```python
from build123d import *

# Parameters (mm, degrees)
SKETCH_1_R      = 2.5
EXTRUDE_1_DEPTH = 3


with BuildPart() as part:
    # 草图1 → 凸台-拉伸1 (new body)
    with BuildSketch(Plane(origin=(0, 0, 0), x_dir=(1, 0, 0), z_dir=(0, 1, 0))):
        with BuildLine():
            ThreePointArc((19, -6), (24.605034154, -2.140932539), (23, 4.472135955))
            Line((23, 4.472135955), (23, 10))
            ThreePointArc((23, 10), (19, 14), (15, 10))
            Line((15, 10), (15, 6))
            Line((15, 6), (0, 6))
            ThreePointArc((0, 6), (-6, 0), (0, -6))
            Line((0, -6), (19, -6))
        make_face()
        with BuildLine():
            ThreePointArc((0.315789474, -3.987515142), (-4, 0), (0.315789474, 3.987515142))
            Line((0.315789474, 3.987515142), (19.197368421, 2.492196964))
            ThreePointArc((19.197368421, 2.492196964), (21.5, 0), (19.197368421, -2.492196964))
            Line((19.197368421, -2.492196964), (0.315789474, -3.987515142))
        make_face(mode=Mode.SUBTRACT)
        with Locations(Location((19, 10, 0), (0, 0, 270))):
            Circle(SKETCH_1_R, mode=Mode.SUBTRACT)
    extrude(amount=EXTRUDE_1_DEPTH)


solid = part.part
```
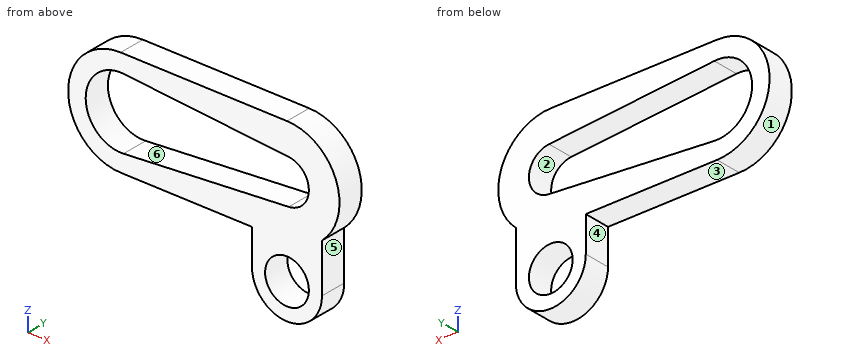
Geometry check sheet. Reference: the model listing, model coordinates, mm. Face numbers are marked on the shaded views. A direction names the side the tool comes from. Round coordinates to 2 decimals unless told otherwise and drop trailing zeros. Order: outer loops, then holes, each group sorted by start corner. A loop starts at its lowest first (then second) coordinate and runs counter-clockwise, first axis right, second up. Notation, with made-up numbers: M 86,-33.5 L 139,-33.5 A22 cw 139,-22.5 Z; hole C 21.5,6 d1. An arc over 180 degrees is marked long. Answer as CSV lines item,"result".
1) Sectioned sample at D-D on z = -7. Record the cut outline in (x, y).
Entries:
outline,"M 15,0 L 23,0 L 23,3 L 15,3 Z"
2) Tool access check on the marked faces 4, 5 and 6. Record the directions out of +Z, -Z, +X, -X, +Y, -Y that give a thin tool (end or side, any length) a straight path to the whole face; none if there is none.
Entries:
face 4,"-Z, -X, +Y, -Y"
face 5,"-Z, +X, +Y, -Y"
face 6,"+Y, -Y"
3) Sectioned sample at B-B on y = 2.65. Record the cut outline in (x, z).
Entries:
outline,"M 0,-6 L 15,-6 L 15,-10 A4 ccw 23,-10 L 23,-4.47 A6 ccw 19,6 L 0,6 A6 ccw Z; hole M 0.32,-3.99 L 19.2,-2.49 A2.5 ccw 19.2,2.49 L 0.32,3.99 A4 ccw long Z; hole C 19,-10 d5"
4) Mould release check, pull along Z, two halves, no side actions. Record for the marked faces 1, 2 and 3: +Z half, -Z half, draft (parallel to the pull), parting line (faces both ways), or undercut.
Entries:
face 1,"parting line"
face 2,"undercut"
face 3,"-Z half"
5) Gauge pin test, flat ends, axial feed: pin 1 Ø1.5 at (x, z) = (6.5, -2) entering from -Y; pin 2 Ø1 at (y, z) = (1.5, -1.5) entering from +X; pin 3 Ø12 at (x, z) = (20.5, -4) entering from -Y; pin 4 Ø1.5 at (x, y) = (7, 2) entering from -Z. Record the tip position at first contact, or that the pin passes through.
Entries:
pin 1,"through"
pin 2,"x = 24.92"
pin 3,"y = 0"
pin 4,"z = -6"
6) Thickness scan on probe 1 along X at (y, z) = (0.8, -10); probe 2 along X at (y, z) = (1.05, -6.5); probe 3 along X at (y, z) = (1.55, -11.25). Record the ranges inside material, lowest first. Write a range as [from, to].
Entries:
probe 1,"[15, 16.5], [21.5, 23]"
probe 2,"[15, 23]"
probe 3,"[15.2, 16.83], [21.17, 22.8]"
7) Sectioned sample at C-C on x = -0.5. Record the cut outline in (y, z).
Entries:
outline,"M 0,-5.98 L 3,-5.98 L 3,-3.97 L 0,-3.97 Z; M 0,3.97 L 3,3.97 L 3,5.98 L 0,5.98 Z"
8) Sectioned sample at A-A on z = 0. Record the cut outline in (x, y), and give its area (3 significant figures).
Entries:
outline,"M -6,0 L -4,0 L -4,3 L -6,3 Z; M 21.5,0 L 25,0 L 25,3 L 21.5,3 Z"
area,"16.5 mm2"
